Design review of the part shown in the three views and the two pictorial views. Dimensions are in mm from the part's minimum x, y and z. A direction names the side the tool comes from. Give positions to 0.01 mm unless a question says otherwise; leave off trailing zeros. Loops run counter-clockwise (first coordinate to the right, second up) from the corner with the lowest first, then second, coordinate; pieces in that order, holes last. Notation, with made-up numbers: (-11, -0.5) - (1, -0.5) arc R21 ccw to (1, 22.5) - close; hole circle Ø2 at (19.25, 17.5). An arc over 180 degrees is marked (long way). Answer as a JSON object with one key per item and string values.
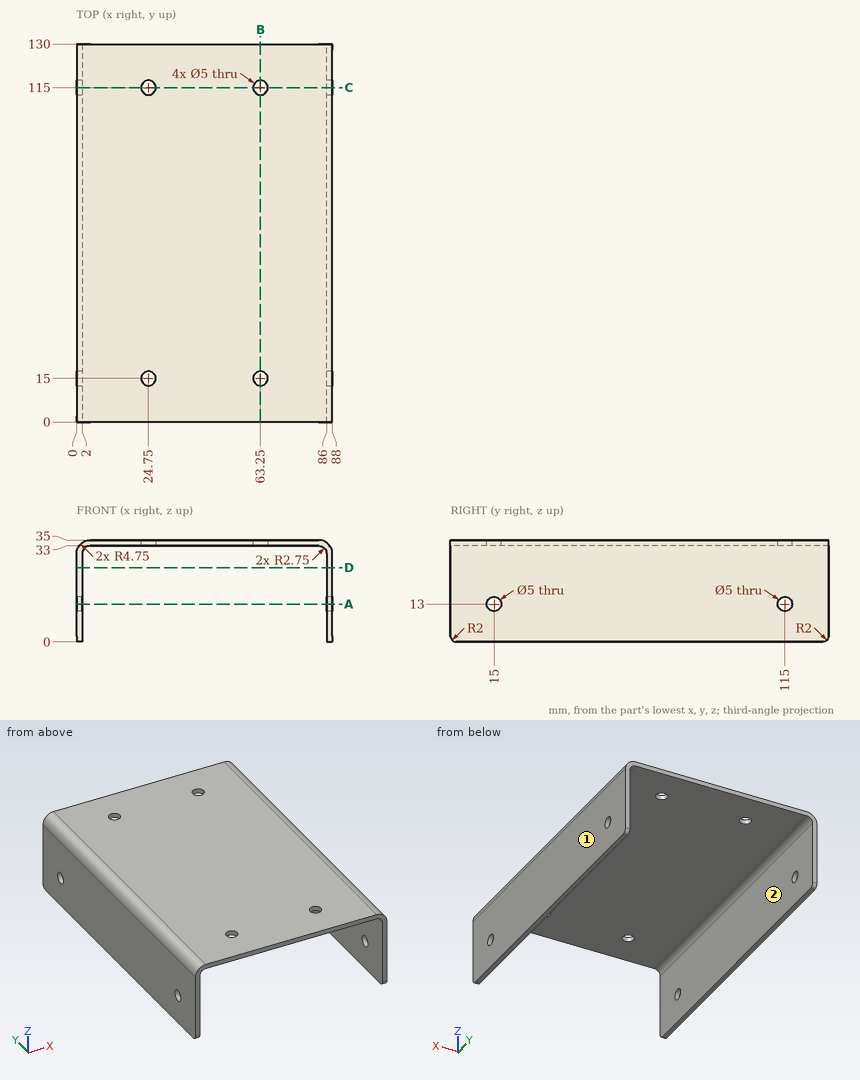
Q1. Consider section D-D, the plane z = 25.5. State the section outline as (x, y) points, plus the area to 3 significant figures.
Results:
{"outline": "(0, 0) - (2, 0) - (2, 130) - (0, 130) - close; (86, 0) - (88, 0) - (88, 130) - (86, 130) - close", "area": "520 mm^2"}
Q2. Consider section C-C, the plane y = 115. State the section outline as (x, z) points, plus the area to 3 significant figures.
Results:
{"outline": "(0, 0) - (2, 0) - (2, 10.5) - (0, 10.5) - close; (0, 15.5) - (2, 15.5) - (2, 30.25) arc R2.75 cw to (4.75, 33) - (22.25, 33) - (22.25, 35) - (4.75, 35) arc R4.75 ccw to (0, 30.25) - close; (27.25, 33) - (60.75, 33) - (60.75, 35) - (27.25, 35) - close; (65.75, 33) - (83.25, 33) arc R2.75 cw to (86, 30.25) - (86, 15.5) - (88, 15.5) - (88, 30.25) arc R4.75 ccw to (83.25, 35) - (65.75, 35) - close; (86, 0) - (88, 0) - (88, 10.5) - (86, 10.5) - close", "area": "262 mm^2"}
Q3. For the marked faces 1 and 2, list the 3-axis set-ups (+Z, -Z, +X, -X, +Y, -Y) from which the entire face can be reached by the end or side of a thin tool; tool diameter is ignored.
Results:
{"face 1": "+Z, -Z, +X, +Y, -Y", "face 2": "-Z, +Y, -Y"}
Q4. Consider section B-B, the plane x = 63.25. State the section outline as (y, z) points, plus the area to 3 significant figures.
Results:
{"outline": "(0, 33) - (12.5, 33) - (12.5, 35) - (0, 35) - close; (17.5, 33) - (112.5, 33) - (112.5, 35) - (17.5, 35) - close; (117.5, 33) - (130, 33) - (130, 35) - (117.5, 35) - close", "area": "240 mm^2"}
Q5. To check wall thickness, follow probe 1 along Y at (x, z) = (63.25, 33.65); probe 2 along X at (y, z) = (114.5, 22); probe 3 along Z at (x, y) = (19, 122.5). State the ranges of each line that lie inside material, in increasing order. Write a range as [from, to].
Results:
{"probe 1": "y = [0, 12.5], [17.5, 112.5], [117.5, 130]", "probe 2": "x = [0, 2], [86, 88]", "probe 3": "z = [33, 35]"}
Q6. Consider section A-A, the plane z = 13. State the section outline as (x, y) points, plus the area to 3 significant figures.
Results:
{"outline": "(0, 0) - (2, 0) - (2, 12.5) - (0, 12.5) - close; (0, 17.5) - (2, 17.5) - (2, 112.5) - (0, 112.5) - close; (0, 117.5) - (2, 117.5) - (2, 130) - (0, 130) - close; (86, 0) - (88, 0) - (88, 12.5) - (86, 12.5) - close; (86, 17.5) - (88, 17.5) - (88, 112.5) - (86, 112.5) - close; (86, 117.5) - (88, 117.5) - (88, 130) - (86, 130) - close", "area": "480 mm^2"}
Q7. Clearance check with flat-ended pins moving along their axes: pin 1 Ø4 at (x, y) = (63.25, 115) entering from +Z; pin 2 Ø23.5 at (x, y) = (24.5, 85.5) entering from -Z. State where each tip first meets the part, or that it passes through.
Results:
{"pin 1": "passes through", "pin 2": "stops at z = 33"}
